Can you work these out from the model? Positions are in its coordinate system, mm. Coordinates: 2 decimals unless noted, no trailing zeros. Write each loop counter-clockwise with the first axis right and the second up, starting at its lowest first coordinate (ties: lowest second). Pieces come first, ordered by that corner, then holes. Notation, with made-up numbers: (-31.75, 61.25) -> (26.25, 61.25) arc R26 cw to (26.25, 87.25) -> close; hole circle Ø7 at (14, 44). An arc over 180 degrees is marked (long way). Use one line per item in the form item = value.
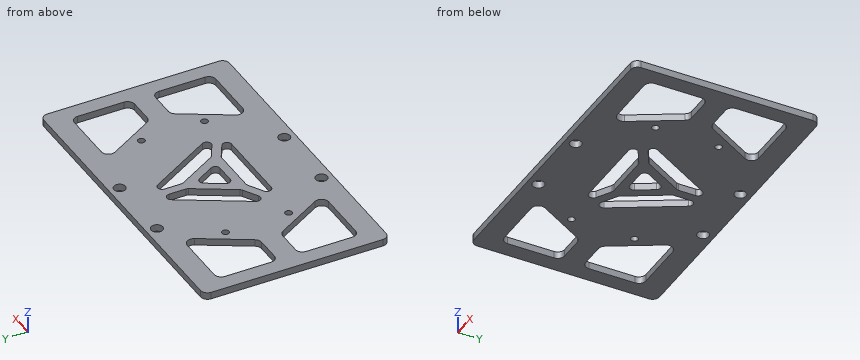
```python
from build123d import *

# Parameters (mm, degrees)
SKETCH_1_W          = 88
SKETCH_1_H          = 53
EXTRUDE_1_DEPTH     = 2
SKETCH_2_R          = 1.65
SKETCH_2_R_2        = 1
CUT_EXTRUDE_1_DEPTH = 10
CUT_EXTRUDE_2_DEPTH = 10
FILLET_1_R          = 1.3
FILLET_4_R          = 2
CUT_EXTRUDE_6_DEPTH = 10
FILLET_5_R          = 2


with BuildPart() as part:
    # 草图1 → 凸台-拉伸1 (new body)
    with BuildSketch(Plane.XY):
        Rectangle(SKETCH_1_W, SKETCH_1_H)
    extrude(amount=EXTRUDE_1_DEPTH)

    # 草图2 → 切除-拉伸1 (cut)
    with BuildSketch(Plane.XY.offset(2)):
        with Locations((7, -23.5)):
            Circle(SKETCH_2_R)
        with Locations((-13, -23.5)):
            Circle(SKETCH_2_R)
        with Locations((-13, 23.5)):
            Circle(SKETCH_2_R)
        with Locations((7, 23.5)):
            Circle(SKETCH_2_R)
        with Locations((22.6, 9)):
            Circle(SKETCH_2_R_2)
        with Locations((22.6, -9)):
            Circle(SKETCH_2_R_2)
        with Locations((-22.6, -9)):
            Circle(SKETCH_2_R_2)
        with Locations((-22.6, 9)):
            Circle(SKETCH_2_R_2)
    extrude(amount=-CUT_EXTRUDE_1_DEPTH, mode=Mode.SUBTRACT)

    # 草图3 → 切除-拉伸2 (cut)
    with BuildSketch(Plane.XY.offset(2)):
        Polygon((0, 5.773502692), (-5, -2.886751346), (5, -2.886751346), align=None)
        Polygon((1.25, 8.608439182), (1.25, 18.608439182), (16.740381057, -8.221687836), (8.080127019, -3.221687836), align=None)
        Polygon((-6.830127019, -5.386751346), (6.830127019, -5.386751346), (15.490381057, -10.386751346), (-15.490381057, -10.386751346), align=None)
        Polygon((-1.25, 8.608439182), (-8.080127019, -3.221687836), (-16.740381057, -8.221687836), (-1.25, 18.608439182), align=None)
    extrude(amount=-CUT_EXTRUDE_2_DEPTH, mode=Mode.SUBTRACT)

    # 圆角1
    fillet_1_edges = [part.edges().sort_by_distance(p)[0] for p in [
        (6.830127019, -5.386751346, 1),
        (15.490381057, -10.386751346, 1),
        (-15.490381057, -10.386751346, 1),
        (-6.830127019, -5.386751346, 1),
        (8.080127019, -3.221687836, 1),
        (1.25, 8.608439182, 1),
        (1.25, 18.608439182, 1),
        (16.740381057, -8.221687836, 1),
        (-8.080127019, -3.221687836, 1),
        (-16.740381057, -8.221687836, 1),
        (-1.25, 18.608439182, 1),
        (-1.25, 8.608439182, 1),
        (5, -2.886751346, 1),
        (-5, -2.886751346, 1),
        (0, 5.773502692, 1),
    ]]
    fillet(fillet_1_edges, radius=FILLET_1_R)

    # 圆角4
    fillet_4_edges = [part.edges().sort_by_distance(p)[0] for p in [
        (44, -26.5, 1),
        (-44, -26.5, 1),
        (-44, 26.5, 1),
        (44, 26.5, 1),
    ]]
    fillet(fillet_4_edges, radius=FILLET_4_R)

    # 草图7 → 切除-拉伸6 (cut)
    with BuildSketch(Plane.XY.offset(2)):
        Polygon((19.5977786, 20.2), (39.5, 20.2), (39.5, 3), (29.52820323, 3), align=None)
        Polygon((29.52820323, -3), (19.5977786, -20.2), (39.5, -20.2), (39.5, -3), align=None)
        Polygon((-39.5, -3), (-29.52820323, -3), (-19.5977786, -20.2), (-39.5, -20.2), align=None)
        Polygon((-39.5, 3), (-29.52820323, 3), (-19.5977786, 20.2), (-39.5, 20.2), align=None)
    extrude(amount=-CUT_EXTRUDE_6_DEPTH, mode=Mode.SUBTRACT)

    # 圆角5
    fillet_5_edges = [part.edges().sort_by_distance(p)[0] for p in [
        (-39.5, 3, 1),
        (-39.5, 20.2, 1),
        (-19.5977786, 20.2, 1),
        (-29.52820323, 3, 1),
        (29.52820323, -3, 1),
        (39.5, -3, 1),
        (39.5, -20.2, 1),
        (19.5977786, -20.2, 1),
        (-39.5, -20.2, 1),
        (-39.5, -3, 1),
        (-29.52820323, -3, 1),
        (-19.5977786, -20.2, 1),
        (29.52820323, 3, 1),
        (19.5977786, 20.2, 1),
        (39.5, 20.2, 1),
        (39.5, 3, 1),
    ]]
    fillet(fillet_5_edges, radius=FILLET_5_R)


solid = part.part
```
Q1. Suppose I cut it at B-B (x = 25). Write out the boundary of the cut face in (y, z).
Return value:
outline = (-26.5, 0) -> (-20.2, 0) -> (-20.2, 2) -> (-26.5, 2) -> close; (-10.84, 0) -> (10.84, 0) -> (10.84, 2) -> (-10.84, 2) -> close; (20.2, 0) -> (26.5, 0) -> (26.5, 2) -> (20.2, 2) -> close
Q2. If I drill on line 1 (Y direction, x = -35, z = 0.2); line 2 (Y direction, x = 22.6, z = 1); line 3 (Y direction, x = 7, z = 1.45), over which ranges is the centre line in solid material (lowest first)? Write a range as from..to.
Return value:
line_1 = -26.5..-20.2, -3..3, 20.2..26.5
line_2 = -26.5..-20.15, -15..-10, -8..8, 10..15, 20.15..26.5
line_3 = -26.5..-25.15, -21.85..-10.39, -5.49..-1.35, 8.65..21.85, 25.15..26.5
Q3. Will these pins go through, and if not, where does the flat tip stop? pin 1 (3 mm diameter, centred on x = 7, y = -23.5, fed in from +Z); pin 2 (1.5 mm diameter, centred on x = -22, y = 1.5, fed in from -Z).
Return value:
pin_1 = through
pin_2 = 0
Q4. Suppose I cut it at C-C (z = 1.4). Give the number of separate pieces and of enclosed holes in the cut face, then the cut area to 3 significant figures.
Return value:
separate_pieces = 1
enclosed_holes = 16
area = 3,250 mm2
Q5. Suppose I cut it at A-A (y = 23.5). Write out the boundary of the cut face in (x, z), then the cut area to 3 significant figures.
Return value:
outline = (-44, 0) -> (-14.65, 0) -> (-14.65, 2) -> (-44, 2) -> close; (-11.35, 0) -> (5.35, 0) -> (5.35, 2) -> (-11.35, 2) -> close; (8.65, 0) -> (44, 0) -> (44, 2) -> (8.65, 2) -> close
area = 163 mm2
